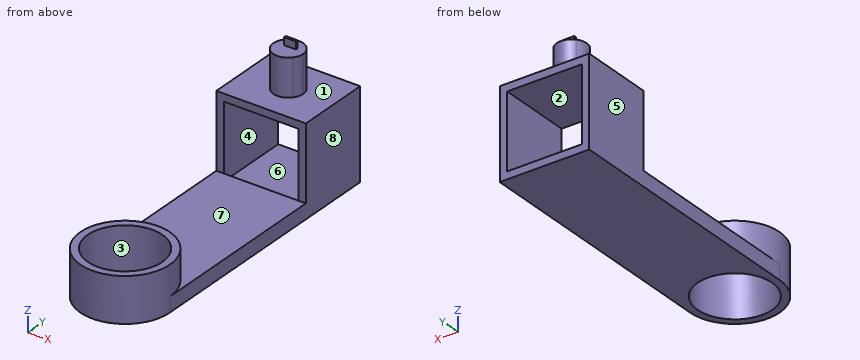
from build123d import *

# Parameters (mm, degrees)
EXTRUDE_1_DEPTH     = 2
SKETCH_4_R          = 6
SKETCH_4_R_2        = 5
EXTRUDE_2_DEPTH     = 6
SKETCH_5_W          = 12
SKETCH_5_H          = 12
EXTRUDE_3_DEPTH     = 10
CUT_EXTRUDE_1_DEPTH = 10
EXTRUDE_4_DEPTH     = 5
SKETCH_9_W          = 1.588517845
SKETCH_9_H          = 0.313853782
EXTRUDE_6_DEPTH     = 1


with BuildPart() as part:
    # 草图1 → 凸台-拉伸1 (new body)
    with BuildSketch(Plane.XY):
        with BuildLine():
            ThreePointArc((-6, 0), (0, 6), (6, 0))
            Line((6, 0), (6, 25))
            Line((6, 25), (-6, 25))
            Line((-6, 25), (-6, 0))
        make_face()
    extrude(amount=EXTRUDE_1_DEPTH)

    # 草图4 → 凸台-拉伸2 (add)
    with BuildSketch(Plane(origin=(0, 0, 0), x_dir=(-1, 0, 0), z_dir=(0, 0, -1))):
        Circle(SKETCH_4_R)
        Circle(SKETCH_4_R_2, mode=Mode.SUBTRACT)
    extrude(amount=-EXTRUDE_2_DEPTH)

    # 草图5 → 凸台-拉伸3 (add)
    with BuildSketch(Plane(origin=(0, 25, 0), x_dir=(1, 0, 0), z_dir=(0, 1, 0))):
        with Locations((0, -6)):
            Rectangle(SKETCH_5_W, SKETCH_5_H)
    extrude(amount=EXTRUDE_3_DEPTH)

    # 草图6 → 切除-拉伸1 (cut)
    with BuildSketch(Plane(origin=(0, 35, 0), x_dir=(1, 0, 0), z_dir=(0, 1, 0))):
        Polygon((5, -1), (-5, -1), (5, -11), align=None)
        Polygon((5, -11), (-5, -1), (-5, -11), align=None)
    extrude(amount=-CUT_EXTRUDE_1_DEPTH, mode=Mode.SUBTRACT)

    # 草图7 → 凸台-拉伸4 (add)
    with BuildSketch(Plane.XY.offset(12)):
        with BuildLine():
            ThreePointArc((2, 30), (0.680850528, 31.880543155), (-1.536442559, 31.280368799))
            Line((-1.536442559, 31.280368799), (1.536442559, 28.719631201))
            ThreePointArc((1.536442559, 28.719631201), (1.880543155, 29.319149472), (2, 30))
        make_face()
        with BuildLine():
            Line((1.536442559, 28.719631201), (-1.536442559, 31.280368799))
            ThreePointArc((-1.536442559, 31.280368799), (-1.280368799, 28.463557441), (1.536442559, 28.719631201))
        make_face()
    extrude(amount=EXTRUDE_4_DEPTH)

    # 草图9 → 凸台-拉伸6 (add)
    with BuildSketch(Plane.XY.offset(17)):
        with Locations((-0.002943276, 30.476616651)):
            Rectangle(SKETCH_9_W, SKETCH_9_H)
    extrude(amount=EXTRUDE_6_DEPTH)


solid = part.part
Read the model definition and answer for the solid it produces. Units are mm, in the model's axes. Face numbers are marked on the shaded views. A direction names the side the tool comes from. Give positions to 0.01 mm unless a question says otherwise; leave off trailing zeros. Write each loop counter-clockwise with the first axis right and the second up, starting at its lowest first coordinate (ties: lowest second). Pieces come first, ordered by that corner, then holes. Notation, with made-up numbers: M 8,23.5 L 15,23.5 A17 cw 15,40.5 Z; hole C -12.5,20 d6. An arc over 180 degrees is marked long. One line per item, written item: value. Start each with the question number.
(1) Find section A-A (z = 9.75). Determine the outline of the cut face in (x, y), plus the area to 3 significant figures.
(2) A tool of negligible diameter and unlimited length cuts with its end or side. For the marked faces 1, 2, 3, 4 and 5, from which of +Z, -Z, +X, -X, +Y, -Y can it reach the whole face along a straight path? Write none if from no direction.
(3) Find section C-C (x = -3). Determine the outline of the cut face in (y, z), plus the area to 3 significant figures.
(4) Find section D-D (z = 12.5). Determine the outline of the cut face in (x, y).
(5) Find section B-B (x = 0). Determine the outline of the cut face in (y, z), plus the area to 3 significant figures.
(6) A flat-ended cylindrical pin translates along its axis: pin 1 Ø0.5 at (x, z) = (-0.5, 17.5) entering from +Y. Find the tip coordinate at first contact, or state that the pin passes through.
(7) Find the intervals of material crossed by line 1 (X direction, y = 32.5, z = 3.75); line 2 (Z direction, x = 4.25, y = 31), in increasing order.
(8) Determine the mould class of the marked faces 6, 7 and 8 for opening direction X: pulls with the +X half, pulls with the -X half, needs draft (parallel to the pull), parting line crosses it, or undercut.
Results below:
1. outline: M -6,25 L -5,25 L -5,35 L -6,35 Z; M 5,25 L 6,25 L 6,35 L 5,35 Z
1. area: 20.0 mm^2
2. face 1: +Z
2. face 2: +Y, -Y
2. face 3: +Z, -Z
2. face 4: +Y
2. face 5: +Z, -Z, -X, +Y, -Y
3. outline: M -5.2,0 L -4,0 L -4,6 L -5.2,6 Z; M 4,0 L 35,0 L 35,1 L 25,1 L 25,2 L 5.2,2 L 5.2,6 L 4,6 Z; M 25,11 L 35,11 L 35,12 L 25,12 Z
3. area: 74.0 mm^2
4. outline: C 0,30 d4
5. outline: M -6,0 L -5,0 L -5,6 L -6,6 Z; M 5,0 L 35,0 L 35,1 L 25,1 L 25,2 L 6,2 L 6,6 L 5,6 Z; M 25,11 L 35,11 L 35,12 L 32,12 L 32,17 L 30.63,17 L 30.63,18 L 30.32,18 L 30.32,17 L 28,17 L 28,12 L 25,12 Z
5. area: 90.3 mm^2
6. pin 1: stops at y = 30.63
7. line 1: x = -6 to -5, 5 to 6
7. line 2: z = 0 to 1, 11 to 12
8. face 6: undercut
8. face 7: needs draft
8. face 8: pulls with the +X half
